Design review of the part built by this model. Coordinates are the model's own, in mm. A direction names the side the tool comes from. Give positions to 0.01 mm unless a question says otherwise; leave off trailing zeros. Order: outer loops, then holes, each group sorted by start corner. A loop starts at its lowest first (then second) coordinate and runs counter-clockwise, first axis right, second up. Notation, with made-up numbers: M -19.75,41 L 24.25,41 A16 ccw 24.25,62 Z; hole C -12.5,46 d4. An arc over 180 degrees is marked long. Put each result on its own line as item: value. Start each with the question number.
Autodesk Inventor part; units mm, degrees
ref_plane "Work Plane1" through (0, 0, -28.575) normal (0, 0, 1) x (1, 0, 0)
ref_plane "Work Plane2" through (0, 6.35, -28.575) normal (0, 1, 0) x (-1, 0, 0)
ref_plane "Work Plane3" through (5.4993, -3.175, -28.575) normal (0.866, -0.5, 0) x (0.5, 0.866, 0)
sketch "Sketch1" plane through (0, 0, 0) normal (0, 0, 1) x (1, 0, 0)
  circle A0 centre (0, 0) radius 6.35
  circle A1 centre (0, 0) radius 3.937
  dimension "d0" = 12.7
  dimension "d1" = 2.413
extrude "Extrusion1" add sketch "Sketch1" against normal blind 304.8
ref_plane "Work Plane1" through (0, 0, -28.575) normal (0, 0, 1) x (1, 0, 0)
sketch "Sketch2" plane through (0, 0, -28.575) normal (0, 0, 1) x (1, 0, 0)
  circle A0 centre (0, 0) radius 6.35
  line L0 (0, 0) -> (5.4993, -3.175) construction
  line L1 (0, 0) -> (0, 6.35) construction
  line L2 (0, 0) -> (-5.4993, -3.175) construction
  dimension "d6" = 120
  dimension "d7" = 120
ref_plane "Work Plane2" through (0, 6.35, -28.575) normal (0, 1, 0) x (-1, 0, 0)
sketch "Sketch3" plane through (0, 6.35, -28.575) normal (0, 1, 0) x (-1, 0, 0)
  circle A0 centre (0, 0) radius 2.3813
  dimension "d8" = 4.7625
extrude "Extrusion2" cut sketch "Sketch3" against normal up to next
ref_plane "Work Plane3" through (5.4993, -3.175, -28.575) normal (0.866, -0.5, 0) x (0.5, 0.866, 0)
sketch "Sketch4" plane through (5.4993, -3.175, -28.575) normal (0.866, -0.5, 0) x (0.5, 0.866, 0)
  circle A0 centre (0, 0) radius 2.3813
  dimension "d11" = 4.7625
extrude "Extrusion3" cut sketch "Sketch4" against normal up to next
ref_plane "Work Plane4" through (-5.4993, -3.175, -28.575) normal (-0.866, -0.5, 0) x (0.5, -0.866, 0)
sketch "Sketch5" plane through (-5.4993, -3.175, -28.575) normal (-0.866, -0.5, 0) x (0.5, -0.866, 0)
  circle A0 centre (0, 0) radius 2.3812
  dimension "d14" = 4.7625
extrude "Extrusion4" cut sketch "Sketch5" against normal up to next
properties part number "transmission tube v1"
1. Consider section A-A on z = -89. Give the boundary of the cut face in (x, y), then the cut area to 3 significant figures.
2. Insertion check: pin 1 (1 mm diameter, centred on y = 2, z = -211, fed in from -X); pin 2 (4 mm diameter, centred on y = -5, z = -245.5, fed in from +X); pin 3 (4 mm diameter, centred on y = -4.5, z = -219.5, fed in from -X). Each pin has a flat end and moves straight along its axis. Give the tip position at first contact, or say it passes through.
3. Machinability: for faces 4 (the cylindrical face through (5.23, -0.48, -29.49)), 5 (the cylindrical face through (-2.2, 4.76, -29.49)), which of the approach directions +Z, -Z, +X, -X, +Y, -Y give a long, thin tool a straight path to every point of the face, cutting with its end or side? Answer none if there is none.
4. To check wall thickness, follow probe 1 along Y at (x, z) = (0, -188); probe 2 along Z at (x, y) = (0, 5.45); probe 3 along Z at (x, y) = (-0.25, 5.5). State the ranges of each line that lie inside material, in increasing order.
5. The part is to be moulded in two halves that separate along Y. For faces 1 (the cylindrical face through (-0.853, -3.843, -150.266)), 2 (the flat face through (-3, -3, -304.8)), 3 (the cylindrical face through (-1.38, -6.2, -150.27)), say which applies: +Y half, -Y half, draft (parallel to the pull), parting line (faces both ways), or undercut.
Returned:
1. outline: C 0,0 d12.7; hole C 0,0 d7.87
1. area: 78.0 mm2
2. pin 1: stops at x = -6.17
2. pin 2: stops at x = 5.6
2. pin 3: stops at x = -5.84
3. face 4: none
3. face 5: +Y
4. probe 1: y = -6.35 to -3.94, 3.94 to 6.35
4. probe 2: z = -304.8 to -30.96, -26.19 to 0
4. probe 3: z = -304.8 to -30.94, -26.21 to 0
5. face 1: undercut
5. face 2: draft
5. face 3: parting line
